from build123d import *

# Parameters (mm, degrees)
BOSS_EXTRUDE1_DEPTH = 15
SKETCH2_R           = 3
CUT_EXTRUDE1_DEPTH  = 51
FILLET1_R           = 3
FILLET2_R           = 3
FILLET3_R           = 3
FILLET4_R           = 3
FILLET5_R           = 3
FILLET6_R           = 3
SKETCH4_W           = 40
SKETCH4_H           = 51
CUT_EXTRUDE2_DEPTH  = 12
SKETCH5_R           = 1
CUT_EXTRUDE3_DEPTH  = 12
FILLET7_R           = 3
FILLET8_R           = 3
SKETCH7_W           = 15
SKETCH7_H           = 22
CUT_EXTRUDE5_DEPTH  = 20
SKETCH9_W           = 15
SKETCH9_H           = 5.5
CUT_EXTRUDE6_DEPTH  = 20
FILLET11_R          = 2
FILLET12_R          = 2
SKETCH11_W          = 12.51
SKETCH11_H          = 51
CUT_EXTRUDE7_DEPTH  = 3
FILLET13_R          = 2
FILLET14_R          = 2


with BuildPart() as part:
    # Sketch1 → Boss-Extrude1 (new body)
    with BuildSketch(Plane(origin=(0, 0, 0), x_dir=(1, 0, 0), z_dir=(0, 1, 0))):
        Polygon((-30, 25.5), (30, 25.5), (30, 18), (15, 18), (15, 13), (30, 13), (30, -13), (15, -13), (15, -18), (30, -18), (30, -25.5), (-30, -25.5), align=None)
    extrude(amount=BOSS_EXTRUDE1_DEPTH)

    # Sketch2 → Cut-Extrude1 (cut)
    with BuildSketch(Plane.XY.offset(25.5)):
        with Locations((25, 7.5)):
            Circle(SKETCH2_R)
    extrude(amount=-CUT_EXTRUDE1_DEPTH, mode=Mode.SUBTRACT)

    # Fillet1
    fillet1_edges = [part.edges().sort_by_distance(p)[0] for p in [
        (30, 15, 21.75),
    ]]
    fillet(fillet1_edges, radius=FILLET1_R)

    # Fillet2
    fillet2_edges = [part.edges().sort_by_distance(p)[0] for p in [
        (30, 15, 0),
    ]]
    fillet(fillet2_edges, radius=FILLET2_R)

    # Fillet3
    fillet3_edges = [part.edges().sort_by_distance(p)[0] for p in [
        (30, 15, -21.75),
    ]]
    fillet(fillet3_edges, radius=FILLET3_R)

    # Fillet4
    fillet4_edges = [part.edges().sort_by_distance(p)[0] for p in [
        (30, 0, 21.75),
    ]]
    fillet(fillet4_edges, radius=FILLET4_R)

    # Fillet5
    fillet5_edges = [part.edges().sort_by_distance(p)[0] for p in [
        (30, 0, 0),
    ]]
    fillet(fillet5_edges, radius=FILLET5_R)

    # Fillet6
    fillet6_edges = [part.edges().sort_by_distance(p)[0] for p in [
        (30, 0, -21.75),
    ]]
    fillet(fillet6_edges, radius=FILLET6_R)

    # Sketch4 → Cut-Extrude2 (cut)
    with BuildSketch(Plane(origin=(0, 15, 0), x_dir=(1, 0, 0), z_dir=(0, 1, 0))):
        with Locations((-10, 0)):
            Rectangle(SKETCH4_W, SKETCH4_H)
    extrude(amount=-CUT_EXTRUDE2_DEPTH, mode=Mode.SUBTRACT)

    # Sketch5 → Cut-Extrude3 (cut)
    with BuildSketch(Plane(origin=(0, 3, 0), x_dir=(1, 0, 0), z_dir=(0, 1, 0))):
        with Locations(Location((-14.99, 22.46, 0), (0, 0, 270))):
            Circle(SKETCH5_R)
        with Locations(Location((-14.99, -22.46, 0), (0, 0, 270))):
            Circle(SKETCH5_R)
    extrude(amount=-CUT_EXTRUDE3_DEPTH, mode=Mode.SUBTRACT)

    # Fillet7
    fillet7_edges = [part.edges().sort_by_distance(p)[0] for p in [
        (10, 15, 0),
    ]]
    fillet(fillet7_edges, radius=FILLET7_R)

    # Fillet8
    fillet8_edges = [part.edges().sort_by_distance(p)[0] for p in [
        (10, 3, 0),
    ]]
    fillet(fillet8_edges, radius=FILLET8_R)

    # Sketch7 → Cut-Extrude5 (cut)
    with BuildSketch(Plane(origin=(0, 15, 0), x_dir=(1, 0, 0), z_dir=(0, 1, 0))):
        with Locations((22.5, 0)):
            Rectangle(SKETCH7_W, SKETCH7_H)
    extrude(amount=-CUT_EXTRUDE5_DEPTH, mode=Mode.SUBTRACT)

    # Sketch9 → Cut-Extrude6 (cut)
    with BuildSketch(Plane(origin=(0, 15, 0), x_dir=(1, 0, 0), z_dir=(0, 1, 0))):
        with Locations((22.5, 22.75)):
            Rectangle(SKETCH9_W, SKETCH9_H)
        with Locations((22.5, -22.75)):
            Rectangle(SKETCH9_W, SKETCH9_H)
    extrude(amount=-CUT_EXTRUDE6_DEPTH, mode=Mode.SUBTRACT)

    # Fillet11
    fillet11_edges = [part.edges().sort_by_distance(p)[0] for p in [
        (15, 7.5, 25.5),
    ]]
    fillet(fillet11_edges, radius=FILLET11_R)

    # Fillet12
    fillet12_edges = [part.edges().sort_by_distance(p)[0] for p in [
        (15, 7.5, -25.5),
    ]]
    fillet(fillet12_edges, radius=FILLET12_R)

    # Sketch11 → Cut-Extrude7 (cut)
    with BuildSketch(Plane(origin=(0, 3, 0), x_dir=(1, 0, 0), z_dir=(0, 1, 0))):
        with Locations((-23.745, 0)):
            Rectangle(SKETCH11_W, SKETCH11_H)
    extrude(amount=-CUT_EXTRUDE7_DEPTH, mode=Mode.SUBTRACT)

    # Fillet13
    fillet13_edges = [part.edges().sort_by_distance(p)[0] for p in [
        (-17.49, 1.5, 25.5),
    ]]
    fillet(fillet13_edges, radius=FILLET13_R)

    # Fillet14
    fillet14_edges = [part.edges().sort_by_distance(p)[0] for p in [
        (-17.49, 1.5, -25.5),
    ]]
    fillet(fillet14_edges, radius=FILLET14_R)


solid = part.part
Part model, mm, in its own coordinate system. A direction names the side the tool comes from. Round coordinates to 2 decimals unless told otherwise and drop trailing zeros. Loops run counter-clockwise (first coordinate to the right, second up) from the corner with the lowest first, then second, coordinate; pieces in that order, holes last. Notation, with made-up numbers: (10, 32) - (52, 32) arc R20 cw to (52, 62) - close; hole circle Ø10 at (41.25, 28.25). An arc over 180 degrees is marked (long way). Answer as a JSON object with one key per item and string values.
Item 1: Pin check, flat tips, straight feed: pin 1 (4.5 mm diameter, centred on x = 23.5, y = 10, fed in from +Z); pin 2 (7.5 mm diameter, centred on x = 23, y = 10, fed in from -Z); pin 3 (19.5 mm diameter, centred on x = -1, z = 1.5, fed in from +Y); pin 4 (1.8 mm diameter, centred on x = -14.99, z = -22.46, fed in from +Y). Stop position of each tip, or through.
Output:
{"pin 1": "z = 20", "pin 2": "z = -20", "pin 3": "y = 3.56", "pin 4": "through"}
Item 2: Wall check: L1, parallel to Z at x = 27.5, y = 13.75; L2, parallel to Y at x = 25, z = -12.05; L3, parallel to Y at x = -10, z = 14. Give the ranges that are in metal, low to high.
Output:
{"L1": "-20 to -18, -13 to -11, 11 to 13, 18 to 20", "L2": "0 to 4.5, 10.5 to 15", "L3": "0 to 3"}
Item 3: Band-saw the part on B-B on x = 25. State how many separate pieces and enclosed holes the cut face has, plus the area to 3 significant figures.
Output:
{"separate pieces": "8", "enclosed holes": "0", "area": "72.0 mm2"}
Item 4: Band-saw the part on A-A on z = 22.46. List the corners of the cut face in (x, y).
Output:
{"outline": "(-17.49, 0) - (-15.99, 0) - (-15.99, 3) - (-17.49, 3) - close; (-13.99, 0) - (15, 0) - (15, 15) - (13, 15) arc R3 ccw to (10, 12) - (10, 6) arc R3 cw to (7, 3) - (-13.99, 3) - close"}
Item 5: Pull direction X, two halves, no side cores. Call faces 6 (the face through (22, 7.6, 12)), 7 (the face through (29.1, 0.86, -18.99)), 8 (the face through (2, 2, 25.5)): pulls with the +X half, pulls with the -X half, needs draft (parallel to the pull), parting line crosses it, or undercut.
Output:
{"face 6": "undercut", "face 7": "pulls with the +X half", "face 8": "needs draft"}
Item 6: Tool access for faces 1 (the face through (2, 2, -25.5)), 2 (the face through (15, 8, 22)), 3 (the face through (-5, 3, 0)), 4 (the face through (30, 7, 12)), 5 (the face through (21, 8, -11)): list every direction of +Z, -Z, +X, -X, +Y, -Y with a clear straight run to the whole face (end or side of a thin tool).
Output:
{"face 1": "-Z, +X, -X, +Y, -Y", "face 2": "+Z, +X, +Y, -Y", "face 3": "+Z, -Z, -X, +Y", "face 4": "+Z, -Z, +X, +Y, -Y", "face 5": "+X, +Y, -Y"}
Item 7: Band-saw the part on D-D on z = 8.5. List the corners of the cut face in (x, y).
Output:
{"outline": "(-17.49, 0) - (15, 0) - (15, 15) - (13, 15) arc R3 ccw to (10, 12) - (10, 6) arc R3 cw to (7, 3) - (-17.49, 3) - close"}
